from build123d import *

# Parameters (mm, degrees)
PAD_DEPTH       = 60
SKETCH004_R     = 2.25
POCKET002_DEPTH = 10
POCKET_DEPTH    = 2


with BuildPart() as part:
    # Sketch → Pad (new body)
    with BuildSketch(Plane.XZ):
        Polygon((-40, 0), (-20, 0), (-20, -15), (20, -15), (20, 0), (40, 0), (40, -10), (30, -10), (30, -25), (-30, -25), (-30, -10), (-40, -10), align=None)
    extrude(amount=PAD_DEPTH)

    # Sketch004 (on DatumPlane) → Pocket002 (cut)
    with BuildSketch(Plane.XY.offset(-10)):
        with Locations((-35, -10)):
            Circle(SKETCH004_R)
        with Locations((35, -10)):
            Circle(SKETCH004_R)
        with Locations((-35, -30)):
            Circle(SKETCH004_R)
        with Locations((35, -30)):
            Circle(SKETCH004_R)
        with Locations((-35, -50)):
            Circle(SKETCH004_R)
        with Locations((-35, -70)):
            Circle(SKETCH004_R)
        with Locations((35, -50)):
            Circle(SKETCH004_R)
        with Locations((35, -70)):
            Circle(SKETCH004_R)
    extrude(amount=POCKET002_DEPTH, mode=Mode.SUBTRACT)

    # Sketch005 (on DatumPlane) → Pocket (cut)
    with BuildSketch(Plane.XY.offset(-10)):
        Polygon((39.041452, -10), (37.020726, -6.5), (32.979274, -6.5), (30.958548, -10), (32.979274, -13.5), (37.020726, -13.5), align=None)
        Polygon((39.041452, -30), (37.020726, -26.5), (32.979274, -26.5), (30.958548, -30), (32.979274, -33.5), (37.020726, -33.5), align=None)
        Polygon((39.041452, -50), (37.020726, -46.5), (32.979274, -46.5), (30.958548, -50), (32.979274, -53.5), (37.020726, -53.5), align=None)
        Polygon((39.041452, -70), (37.020726, -66.5), (32.979274, -66.5), (30.958548, -70), (32.979274, -73.5), (37.020726, -73.5), align=None)
    extrude(amount=POCKET_DEPTH, mode=Mode.SUBTRACT)


solid = part.part
Build history of the part. All positions in model axes, mm. A direction names the side the tool comes from. Give positions to 0.01 mm unless a question says otherwise; leave off trailing zeros. Write each loop counter-clockwise with the first axis right and the second up, starting at its lowest first coordinate (ties: lowest second). Pieces come first, ordered by that corner, then holes. Notation, with made-up numbers: (40.5, -6.5) - (72.5, -6.5) arc R5 ccw to (72.5, -0.5) - close; hole circle Ø1 at (-39.5, 19). An arc over 180 degrees is marked (long way). Use one line per item in the form item = value. Start each with the question number.
1. Band-saw the part on D-D on x = -1. Write the cut outline in (y, z), plus the area to 3 significant figures.
2. Band-saw the part on A-A on z = -5.5. Write the cut outline in (x, y), plus the area to 3 significant figures.
3. Drop flat-ended pins along their axis: pin 1 Ø5.5 at (x, y) = (34, -50.5) entering from -Z; pin 2 Ø4 at (x, y) = (35, -50) entering from +Z; pin 3 Ø10 at (y, z) = (-50, -21) entering from +X; pin 4 Ø3 at (x, y) = (11.5, -47) entering from +Z. Give the stop position or say it passes through.
4. Band-saw the part on B-B on z = -11. Write the cut outline in (x, y), plus the area to 3 significant figures.
5. Two-plate mould, pull along Y, no slides. Class faces 5 (the face through (38, -11.8, -9)), 6 (the face through (1, 0, -18)), 7 (the face through (1, -60, -18)), 8 (the face through (38.045, -48.274, -9.014)): released by +Y, released by -Y, zero draft, split by the parting line, or undercut.
6. 3-axis set-ups, long thin cutter, end or side, ignore diameter. For faces 1 (the face through (30.6, -29.6, -10)), 2 (the face through (35, -26.5, -9)), 3 (the face through (20, -30, -8)), 4 (the face through (-30, -30, -18)): which of +Z, -Z, +X, -X, +Y, -Y reach the whole face in a straight line?
7. Probe line 1 (Y direction, x = 35, z = -6.5); line 2 (X direction, y = -43, z = -12.5); line 3 (X direction, y = -45, z = -4.5). List the from-to ranges inside material, lowest first. Write a range as [from, to].
8. Band-saw the part on C-C on y = -20.5. Write the cut outline in (x, z).
Conclusion:
q1.outline = (-60, -25) - (0, -25) - (0, -15) - (-60, -15) - close
q1.area = 600 mm²
q2.outline = (-40, -60) - (-20, -60) - (-20, 0) - (-40, 0) - close; (20, -60) - (40, -60) - (40, 0) - (20, 0) - close; hole circle Ø4.5 at (-35, -50); hole circle Ø4.5 at (-35, -30); hole circle Ø4.5 at (-35, -10); hole circle Ø4.5 at (35, -50); hole circle Ø4.5 at (35, -30); hole circle Ø4.5 at (35, -10)
q2.area = 2,300 mm²
q3.pin_1 = -10
q3.pin_2 = through
q3.pin_3 = 30
q3.pin_4 = -15
q4.outline = (-30, -60) - (-20, -60) - (-20, 0) - (-30, 0) - close; (20, -60) - (30, -60) - (30, 0) - (20, 0) - close
q4.area = 1,200 mm²
q5.face_5 = undercut
q5.face_6 = released by +Y
q5.face_7 = released by -Y
q5.face_8 = undercut
q6.face_1 = -Z, +X, +Y, -Y
q6.face_2 = -Z
q6.face_3 = +Z, +Y, -Y
q6.face_4 = -Z, -X, +Y, -Y
q7.line_1 = [-60, -52.25], [-47.75, -32.25], [-27.75, -12.25], [-7.75, 0]
q7.line_2 = [-30, -20], [20, 30]
q7.line_3 = [-40, -20], [20, 40]
q8.outline = (-40, -10) - (-30, -10) - (-30, -25) - (30, -25) - (30, -10) - (40, -10) - (40, 0) - (20, 0) - (20, -15) - (-20, -15) - (-20, 0) - (-40, 0) - close
